Check sheet for the drawn part. Datum: minimum x, y, z corner. Units: mm. A direction names the side the tool comes from. Round coordinates to 2 decimals unless told otherwise and drop trailing zeros. Write each loop counter-clockwise with the first axis right and the second up, starting at its lowest first coordinate (ties: lowest second). Pieces come first, ordered by that corner, then holes.
Item 1: Go/stop test with flat-tipped pins: pin 1 Ø1 at (y, z) = (18, 1) entering from -X; pin 2 Ø1 at (x, y) = (9.5, 15.5) entering from -Z. Record where each tip stops, or that it passes through.
Item 2: Release check for a two-part mould opening along Z. For the marked faces 3, 4 and 5 record: +Z half, -Z half, draft (parallel to the pull), parting line (faces both ways), or undercut.
Item 3: Cross-section at B-B on y = 15.25. Enter the section's corners in (x, z), plus the area to 3 significant figures.
Item 4: Cross-section at D-D on x = 10. Enter the section's corners in (y, z), plus the area to 3 significant figures.
Item 5: Material ranges on line 1 (Z direction, x = 28, y = 19.75); line 2 (Y direction, x = 38, z = 26.75); line 3 (Z direction, x = 9, y = 24.25), recorded low to high.
Item 6: Cross-section at C-C on z = 16.5. Enter the section's corners in (x, y).
Item 7: Tool access check on the marked faces 1 and 2. Record the directions out of +Z, -Z, +X, -X, +Y, -Y that give a thin tool (end or side, any length) a straight path to the whole face; none if there is none.
Item 8: Cross-section at A-A on x = 40.5. Enter the section's corners in (y, z).
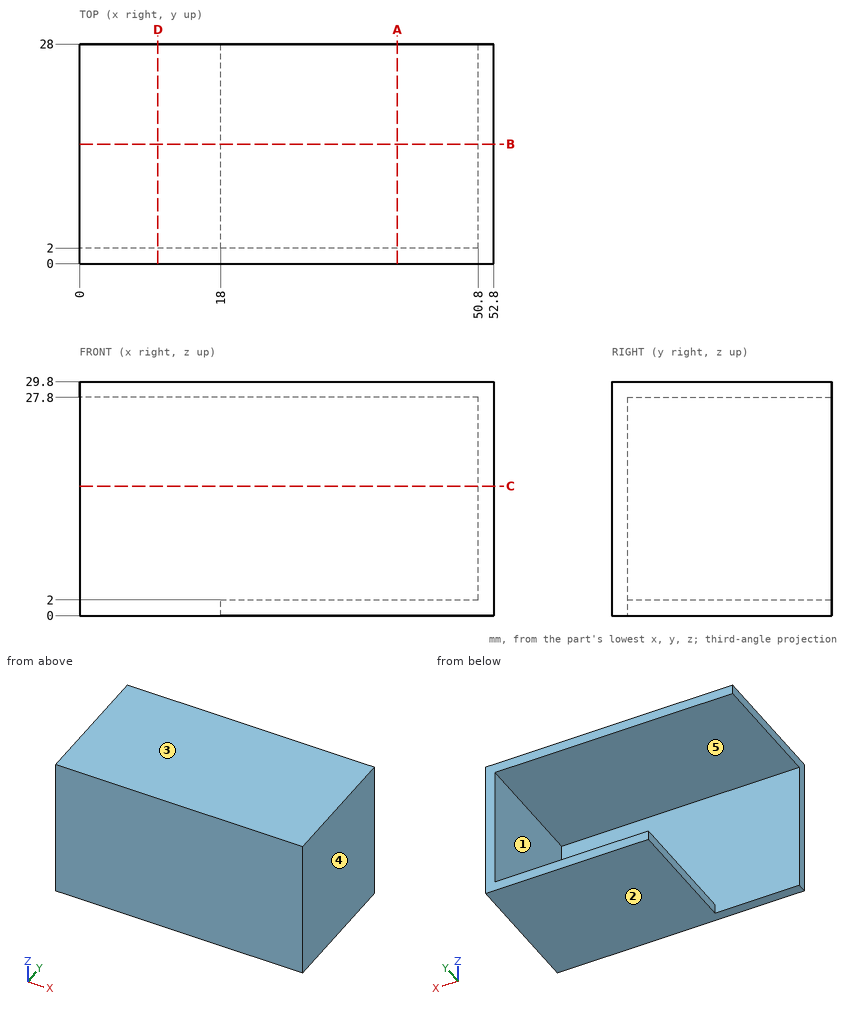
Response values:
1. pin 1: stops at x = 18
1. pin 2: stops at z = 27.8
2. face 3: +Z half
2. face 4: draft
2. face 5: undercut
3. outline: (0, 27.8) - (50.8, 27.8) - (50.8, 2) - (18, 2) - (18, 0) - (52.8, 0) - (52.8, 29.8) - (0, 29.8) - close
3. area: 227 mm2
4. outline: (0, 0) - (2, 0) - (2, 27.8) - (28, 27.8) - (28, 29.8) - (0, 29.8) - close
4. area: 112 mm2
5. line 1: z = 0 to 2, 27.8 to 29.8
5. line 2: y = 0 to 2
5. line 3: z = 27.8 to 29.8
6. outline: (0, 0) - (52.8, 0) - (52.8, 28) - (50.8, 28) - (50.8, 2) - (0, 2) - close
7. face 1: -X, +Y
7. face 2: -Z, +X, -X, +Y, -Y
8. outline: (0, 0) - (28, 0) - (28, 2) - (2, 2) - (2, 27.8) - (28, 27.8) - (28, 29.8) - (0, 29.8) - close
